Source: CAD feature listing. Evaluate the final solid. Frame: model axes, mm. A direction names the side the tool comes from. Coordinates: 2 decimals unless noted, no trailing zeros. Order: outer loops, then holes, each group sorted by start corner. A loop starts at its lowest first (then second) coordinate and runs counter-clockwise, first axis right, second up.
```python
from build123d import *

# Parameters (mm, degrees)
SKETCH_W     = 28
SKETCH_H     = 8
PAD_DEPTH    = 4
PAD001_DEPTH = 150
SKETCH002_R  = 1.25
POCKET_DEPTH = 1.8


with BuildPart() as part:
    # Sketch → Pad (new body)
    with BuildSketch(Plane.XY):
        with Locations((-14, 0)):
            Rectangle(SKETCH_W, SKETCH_H)
    pad = extrude(amount=PAD_DEPTH)

    # Sketch001 (on Face6 of Pad) → Pad001 (join)
    with BuildSketch(Plane.XY.offset(4)):
        Polygon((-22.5, 0.9), (-25.5, 0.9), (-25.5, 4), (-28, 4), (-28, -4), (-25.5, -4), (-25.5, -0.9), (-22.5, -0.9), (-22.5, -4), (0, -4), (0, 4), (-22.5, 4), align=None)
    pad001 = extrude(amount=PAD001_DEPTH)

    # Sketch002 (on Face14 of Pad001) → Pocket (cut)
    with BuildSketch(Plane(origin=(0, 0.9, 0), x_dir=(-1, 0, 0), z_dir=(0, 1, 0))):
        with Locations((24, 151)):
            Circle(SKETCH002_R)
    pocket = extrude(amount=-POCKET_DEPTH, mode=Mode.SUBTRACT)

    # Mirrored: Pad, Pad001, Pocket across Sketch V_Axis
    add(pad.mirror(Plane(origin=(0, 0, 0), x_dir=(0, 0, 1), z_dir=(1, 0, 0))))
    add(pad001.mirror(Plane(origin=(0, 0, 0), x_dir=(0, 0, 1), z_dir=(1, 0, 0))))
    add(pocket.mirror(Plane(origin=(0, 0, 0), x_dir=(0, 0, 1), z_dir=(1, 0, 0))), mode=Mode.SUBTRACT)


solid = part.part
```
Q1. Pull-direction query (X, two-part tool) for faces 4 (the flat face through (0, 0, 0)), 5 (the flat face through (28, 0, 76)), 6 (the flat face through (-22.5, -2, 78)); classes: pulls with the +X half, pulls with the -X half, needs draft (parallel to the pull), parting line crosses it, or undercut.
Solutions:
face 4: needs draft
face 5: pulls with the +X half
face 6: undercut
Q2. Section query A-A on z = 116.5. Output: boundary loops of the cut face in (x, y), plus the area to 3 significant figures.
Solutions:
outline: (-28, -4) - (-25.5, -4) - (-25.5, -0.9) - (-22.5, -0.9) - (-22.5, -4) - (22.5, -4) - (22.5, -0.9) - (25.5, -0.9) - (25.5, -4) - (28, -4) - (28, 4) - (25.5, 4) - (25.5, 0.9) - (22.5, 0.9) - (22.5, 4) - (-22.5, 4) - (-22.5, 0.9) - (-25.5, 0.9) - (-25.5, 4) - (-28, 4) - close
area: 411 mm2
Q3. Section query B-B on y = 2.5. Output: boundary loops of the cut face in (x, z).
Solutions:
outline: (-28, 0) - (28, 0) - (28, 154) - (25.5, 154) - (25.5, 4) - (22.5, 4) - (22.5, 154) - (-22.5, 154) - (-22.5, 4) - (-25.5, 4) - (-25.5, 154) - (-28, 154) - close
Q4. Material intervals for line 1 along X through (y, z) = (3, 147); line 2 along X through (y, z) = (0.5, 151); line 3 along Z through (x, y) = (24, 0.35), sorted ascending.
Solutions:
line 1: x = -28 to -25.5, -22.5 to 22.5, 25.5 to 28
line 2: x = -28 to -25.25, -22.75 to 22.75, 25.25 to 28
line 3: z = 0 to 149.75, 152.25 to 154
Q5. Set-up query: faces 1 (the flat face through (-25.5, -2, 78)), 2 (the flat face through (-28, 0, 76)), 3 (the flat face through (25.5, 2, 78)). Return all of +Z, -Z, +X, -X, +Y, -Y with unobstructed straight access to the full face (end or side cutting, diameter ignored); none if empty.
Solutions:
face 1: +Z, -Y
face 2: +Z, -Z, -X, +Y, -Y
face 3: +Z, +Y
Q6. Pin query (flat end, axial travel): P1, Ø1.5, axis at x = -23.5, y = -2, coming from the +Z side; P2, Ø2.5, axis at x = 24, z = 84, coming from the +Y side; P3, Ø2, axis at x = 24, z = 151, coming from the -Y side; P4, Ø2.5, axis at x = -24, z = 73.5, coming from the -Y side. Return the tip coordinate at first contact, or that it passes through.
Solutions:
P1: stops at z = 4
P2: stops at y = 0.9
P3: passes through
P4: stops at y = -0.9
